```python
from build123d import *

# Parameters (mm, degrees)
F0_R     = 1
F1_DEPTH = 1.5


with BuildPart() as f1:
    # F0 (on Right) → F1 (new body)
    with BuildSketch(Plane.YZ):
        Polygon((-2, 0), (0, 0), (0, 24.5), (-2, 24.5), (-2, 26.5), (-10, 26.5), (-10, 24.5), (-18, 24.5), (-18, 26.5), (-24, 26.5), (-24, 24.5), (-31, 12), (-25, 12), (-25, 10), (-31, 10), (-26, 0), (-24, 0), (-24, -2), (-18, -2), (-18, 0), (-10, 0), (-10, -2), (-2, -2), align=None)
        with Locations((-13, 10)):
            Circle(F0_R, mode=Mode.SUBTRACT)
    extrude(amount=F1_DEPTH)


solid = f1.part
```
Work out the finished part from the listing and answer in its coordinate system (mm). A direction names the side the tool comes from. Coordinates: 2 decimals unless noted, no trailing zeros. Loops run counter-clockwise (first coordinate to the right, second up) from the corner with the lowest first, then second, coordinate; pieces in that order, holes last. Notation, with made-up numbers: (-36, 69.25) - (0, 69.25) arc R24 cw to (0, 95.25) - close; hole circle Ø8 at (1.5, 5.25). An arc over 180 degrees is marked (long way). Use a Markdown table: item, result.
Item 1: Consider probe 1 along Z at (x, y) = (0.7, -13); probe 2 along Y at (x, z) = (0.7, 9.5); probe 3 along Z at (x, y) = (1.45, -0.5). Determine where each line is inside the solid, lowest interval first. Write a range as from..to.
Evaluation:
| item | result |
|---|---|
| probe 1 | z = 0..9, 11..24.5 |
| probe 2 | y = -30.75..-13.87, -12.13..0 |
| probe 3 | z = 0..24.5 |
Item 2: For faces 4 (the flat face through (1, -25, 11)), 5 (the flat face through (1, -2, 25)), 6 (the flat face through (1, -25, 0)), determine the directions among +Z, -Z, +X, -X, +Y, -Y from which every point of the face is accessible in a straight line to the end or side of a thin tool.
Evaluation:
| item | result |
|---|---|
| face 4 | +X, -X, -Y |
| face 5 | +Z, +X, -X, +Y |
| face 6 | -Z, +X, -X, -Y |
Item 3: The mould has two halves that part along Z. Classify faces 1 (the flat face through (1, -1, 0)), 2 (the flat face through (1, -21, 26.5)), 3 (the flat face through (1, -28, 10)): +Z half, -Z half, draft (parallel to the pull), parting line (faces both ways), or undercut.
Evaluation:
| item | result |
|---|---|
| face 1 | -Z half |
| face 2 | +Z half |
| face 3 | undercut |
Item 4: Find section A-A, the plane y = -13. Determine the outline of the cut face in (x, z).
Evaluation:
| item | result |
|---|---|
| outline | (0, 0) - (1.5, 0) - (1.5, 9) - (0, 9) - close; (0, 11) - (1.5, 11) - (1.5, 24.5) - (0, 24.5) - close |
Item 5: Find section D-D, the plane z = 20.25. Determine the outline of the cut face in (x, y).
Evaluation:
| item | result |
|---|---|
| outline | (0, -26.38) - (1.5, -26.38) - (1.5, 0) - (0, 0) - close |
Item 6: Find section C-C, the plane z = 16.5. Determine the outline of the cut face in (x, y).
Evaluation:
| item | result |
|---|---|
| outline | (0, -28.48) - (1.5, -28.48) - (1.5, 0) - (0, 0) - close |
Item 7: Find section B-B, the plane x = 0.5. Determine the outline of the cut face in (y, z).
Evaluation:
| item | result |
|---|---|
| outline | (-31, 10) - (-26, 0) - (-24, 0) - (-24, -2) - (-18, -2) - (-18, 0) - (-10, 0) - (-10, -2) - (-2, -2) - (-2, 0) - (0, 0) - (0, 24.5) - (-2, 24.5) - (-2, 26.5) - (-10, 26.5) - (-10, 24.5) - (-18, 24.5) - (-18, 26.5) - (-24, 26.5) - (-24, 24.5) - (-31, 12) - (-25, 12) - (-25, 10) - close; hole circle Ø2 at (-13, 10) |
Item 8: Given pin 1 Ø0.8 at (x, z) = (0.5, -1) entering from -Y; pin 2 Ø1.6 at (y, z) = (-13, 10) entering from +X, each flat-ended and moving along its own axis, determine where each tip first touches the part or whether it passes through.
Evaluation:
| item | result |
|---|---|
| pin 1 | stops at y = -24 |
| pin 2 | passes through |
